```python
from build123d import *

# Parameters (mm, degrees)
F0_R        = 15.875
F0_R_2      = 14.2875
F1_DEPTH    = 44.45
F2_R        = 17.145
F2_R_2      = 14.2875
F3_DEPTH    = 16.51
F5_S5_R     = 15.875
F5_T6_DEPTH = 26


# Not quite as in the source:
# - a fillet or chamfer that OpenCascade refuses, or shapes differently, is made with other operations: its cross-section is extruded or revolved along the edge and cut away or added


with BuildPart() as f1:
    # F0 (on Top) → F1 (new body, symmetric)
    with BuildSketch(Plane.XY):
        Circle(F0_R)
        Circle(F0_R_2, mode=Mode.SUBTRACT)
    extrude(amount=F1_DEPTH, both=True)

    # F2 (on face) → F3 (join)
    with BuildSketch(Plane.XY.offset(44.45)):
        Circle(F2_R)
        Circle(F2_R_2, mode=Mode.SUBTRACT)
    extrude(amount=F3_DEPTH)

    # F4: chamfer of 3.81 x 8.89 on 1 edges, made by hand

    # F4_s1 → F4_t2 (revolve, cut)
    with BuildSketch(Plane.XZ):
        Polygon((17.145, 52.07), (13.335, 60.96), (17.145, 60.96), align=None)
    revolve(axis=Axis((0, 0, 60.96), (0, 0, 1)), mode=Mode.SUBTRACT)

    # F5: chamfer of 1.524 on 1 edges, made by hand


with BuildPart() as f5_tool2:
    # F5_s3 → F5_t4 (revolve)
    with BuildSketch(Plane.XZ):
        Polygon((15.621, 44.45), (17.145, 45.974), (17.145, 44.45), align=None)
    revolve(axis=Axis((0, 0, 44.45), (0, 0, 1)))

    # F5_s5 → F5_t6 (cut, symmetric)
    with BuildSketch(Plane.XY.offset(45.2)):
        Circle(F5_S5_R)
    extrude(amount=F5_T6_DEPTH, both=True, mode=Mode.SUBTRACT)


with BuildPart() as f1_1:
    add(f1.part)

    # F5_t1: cut F5_tool2
    add(f5_tool2.part, mode=Mode.SUBTRACT)


solid = f1_1.part
```
Design review of the part built by this model. Coordinates are the model's own, in mm. Round coordinates to 2 decimals unless told otherwise and drop trailing zeros. Write each loop counter-clockwise with the first axis right and the second up, starting at its lowest first coordinate (ties: lowest second). Pieces come first, ordered by that corner, then holes.
Item 1: Clearance check with flat-ended pins moving along their axes: pin 1 Ø2 at (x, z) = (-4, 32.5) entering from -Y; pin 2 Ø1 at (y, z) = (-9.5, 28) entering from +X; pin 3 Ø1.5 at (x, z) = (2, 43.5) entering from -Y. State where each tip first meets the part, or that it passes through.
Item 2: The part is to be moulded in two halves that separate along Y. For faces 1 (the cylindrical face through (15.14, 4.77, 0.75)), 2 (the cylindrical face through (-14.274, 0.628, 6.421)), 3 (the flat face through (-11.83, 8.31, -44.45)), say which applies: +Y half, -Y half, draft (parallel to the pull), parting line (faces both ways), or undercut.
Item 3: We need section C-C on z = 51. Write out the cut boundary in (x, y) (1 decimal), and give its area (3 significant figures).
Item 4: For probe 1 along Y at (x, z) = (0, 4.5) (1 decimal); probe 2 along Y at (x, z) = (10, 33.5); probe 3 along X at (y, z) = (4.5, -37), list the stretches that pass through material, from the lowest coordinate up.
Returned:
1. pin 1: stops at y = -15.59
1. pin 2: stops at x = 13.08
1. pin 3: stops at y = -15.83
2. face 1: parting line
2. face 2: undercut
2. face 3: draft
3. outline: circle Ø34.3 at (0, 0); hole circle Ø28.6 at (0, 0)
3. area: 282 mm2
4. probe 1: y = -15.9 to -14.3, 14.3 to 15.9
4. probe 2: y = -12.33 to -10.2, 10.2 to 12.33
4. probe 3: x = -15.22 to -13.56, 13.56 to 15.22
